The listing builds one solid part. Answer for the finished solid, in the listing's coordinates (mm). Face numbers are marked on the shaded views. A direction names the side the tool comes from. Coordinates: 2 decimals unless noted, no trailing zeros. Write each loop counter-clockwise with the first axis right and the second up, starting at its lowest first coordinate (ties: lowest second). Pieces come first, ordered by that corner, then holes. Notation, with made-up numbers: M 14.25,29 L 47.25,29 A28 cw 47.25,61 Z; hole C -3,-2.75 d2. An arc over 180 degrees is marked long. Answer as CSV lines item,"result".
```python
from build123d import *

# Parameters (mm, degrees)
SKETCH1_R           = 2.4
BOSS_EXTRUDE1_DEPTH = 13.3
FILLET1_R           = 0.1905


with BuildPart() as part:
    # Sketch1 → Boss-Extrude1 (new body)
    with BuildSketch(Plane(origin=(0, 0, 0), x_dir=(1, 0, 0), z_dir=(0, 1, 0))):
        Circle(SKETCH1_R)
    extrude(amount=BOSS_EXTRUDE1_DEPTH)

    # Sketch2 → Revolve1 (revolve)
    with BuildSketch(Plane.XY):
        with BuildLine():
            Line((-4.55, 13.3), (0, 13.3))
            Line((0, 13.3), (0, 16.2))
            add(Edge.make_bspline(
                [(0, 16.2), (-1.798533353, 16.2), (-3.716538693, 15.437253148), (-4.55, 13.3)],
                knots=[0, 0, 0, 0, 1, 1, 1, 1], degree=3))
        make_face()
    revolve(axis=Axis((0, 13.3, 0), (0, 1, 0)))

    # Fillet1
    fillet1_edges = [part.edges().sort_by_distance(p)[0] for p in [
        (4.55, 13.3, 0),
    ]]
    fillet(fillet1_edges, radius=FILLET1_R)


solid = part.part
```
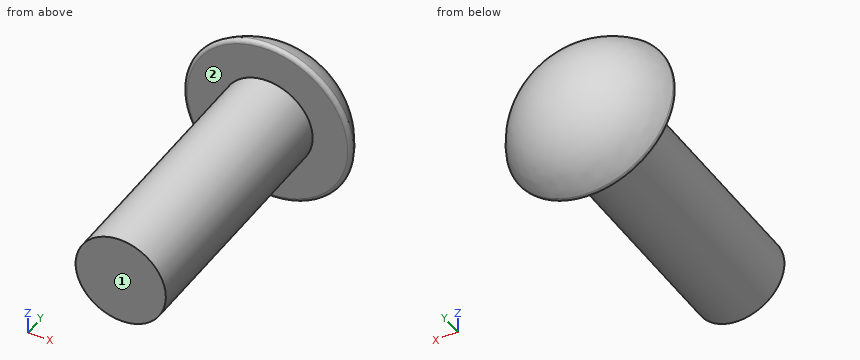
Q1. Flat-ended cylindrical pins translate along their axes: pin 1 Ø3 at (x, z) = (1.5, 0.5) entering from -Y; pin 2 Ø1 at (x, y) = (-2.5, 13.5) entering from -Z; pin 3 Ø3 at (x, y) = (0, 5) entering from -Z; pin 4 Ø2 at (y, z) = (2.5, 0) entering from -X. Find the tip coordinate at first contact, or state that the pin passes through.
Output:
pin 1,"y = 0"
pin 2,"z = -3.98"
pin 3,"z = -2.4"
pin 4,"x = -2.4"
Q2. For the marked faces 1 and 2, determine the directions among +Z, -Z, +X, -X, +Y, -Y from which every point of the face is accessible in a straight line to the end or side of a thin tool.
Output:
face 1,"+Z, -Z, +X, -X, -Y"
face 2,"-Y"
Q3. Find section A-A (y = 10). Give the vertices of the cut face in (x, z).
Output:
outline,"C 0,0 d4.8"
Q4. Straight lines are drawn through the part: line 1 (Z direction, x = 0, y = 12.5); line 2 (Z direction, x = 2.75, y = 13.75); line 3 (X direction, y = 14, z = 0). For each, find the intervals that lie inside material, in ascending order.
Output:
line 1,"-2.4 to 2.4"
line 2,"-3.37 to 3.37"
line 3,"-4.21 to 4.21"
